Build history of the part. All positions in model axes, mm. A direction names the side the tool comes from. Coordinates: 2 decimals unless noted, no trailing zeros. Order: outer loops, then holes, each group sorted by start corner. A loop starts at its lowest first (then second) coordinate and runs counter-clockwise, first axis right, second up. Notation, with made-up numbers: (-26, 45.5) - (-1, 45.5) arc R32 cw to (-1, 80.5) - close; hole circle Ø11 at (45, 39.25). An arc over 180 degrees is marked (long way). One line per item, written item: value.
from build123d import *
from build123d.topology import SkipClean

# Parameters (mm, degrees)
SKETCH1_R               = 5.5
BOSS_EXTRUDE1_DEPTH     = 17
SKETCH2_R               = 10
BOSS_EXTRUDE2_DEPTH     = 5
BOSS_EXTRUDE3_DEPTH     = 3
BOSS_EXTRUDE4_START     = -6.6383
BOSS_EXTRUDE4_DEPTH     = 6.6383
CIRPATTERN1_COUNT       = 4
SKETCH10_R              = 13.301263659
CUT_EXTRUDE3_DEPTH      = 4
CUT_EXTRUDE3_DEPTH_BACK = 23
FILLET1_R               = 2
CUT_EXTRUDE4_DEPTH      = 6
SKETCH12_R              = 5
CUT_EXTRUDE5_DEPTH      = 3


with BuildPart() as part:
    # Sketch1 → Boss-Extrude1 (new body)
    with BuildSketch(Plane(origin=(0, 0, 0), x_dir=(1, 0, 0), z_dir=(0, 1, 0))):
        with Locations(Location((0, 0, 0), (0, 0, 270))):  # turned: the seam where the file's is
            Circle(SKETCH1_R)
    extrude(amount=BOSS_EXTRUDE1_DEPTH)

    # Sketch2 → Boss-Extrude2 (add)
    with BuildSketch(Plane(origin=(0, 17, 0), x_dir=(1, 0, 0), z_dir=(0, 1, 0))):
        with Locations(Location((0, 0, 0), (0, 0, 270))):  # turned: the seam where the file's is
            Circle(SKETCH2_R)
    extrude(amount=BOSS_EXTRUDE2_DEPTH)

    # Sketch4 → Boss-Extrude3 (add)
    with BuildSketch(Plane(origin=(0, 22, 0), x_dir=(1, 0, 0), z_dir=(0, 1, 0))):
        with BuildLine():
            Line((1, 10), (-1, 10))
            Line((-1, 10), (-1, 4.898979486))
            ThreePointArc((-1, 4.898979486), (-3.535533906, 3.535533906), (-4.898979486, 1))
            Line((-4.898979486, 1), (-10, 1))
            Line((-10, 1), (-10, -1))
            Line((-10, -1), (-4.898979486, -1))
            ThreePointArc((-4.898979486, -1), (-3.535533906, -3.535533906), (-1, -4.898979486))
            Line((-1, -4.898979486), (-1, -10))
            Line((-1, -10), (1, -10))
            Line((1, -10), (1, -4.898979486))
            ThreePointArc((1, -4.898979486), (3.535533906, -3.535533906), (4.898979486, -1))
            Line((4.898979486, -1), (10, -1))
            Line((10, -1), (10, 1))
            Line((10, 1), (4.898979486, 1))
            ThreePointArc((4.898979486, 1), (3.535533906, 3.535533906), (1, 4.898979486))
            Line((1, 4.898979486), (1, 10))
        make_face()
    extrude(amount=BOSS_EXTRUDE3_DEPTH)

    # Sketch9 → Boss-Extrude4 (add)
    with BuildSketch(Plane(origin=(0, 0, -10), x_dir=(-1, 0, 0), z_dir=(0, 0, -1)).offset(BOSS_EXTRUDE4_START)):
        Polygon((-1, 25), (-3.701212133, 22), (-1, 22), align=None)
    boss_extrude4 = extrude(amount=BOSS_EXTRUDE4_DEPTH)

    # CirPattern1: Boss-Extrude4 ×4 about axis
    cirpattern1_axis = Axis((0, 0, 0), (0, 1, 0))
    for i in range(1, CIRPATTERN1_COUNT):
        add(boss_extrude4.rotate(cirpattern1_axis, i * 360 / CIRPATTERN1_COUNT))

    # Sketch10 → Cut-Extrude3 (cut, two sides)
    with BuildSketch(Plane(origin=(0, 22, 0), x_dir=(1, 0, 0), z_dir=(0, 1, 0))) as cut_extrude3_sk:
        Circle(SKETCH10_R)
        with BuildLine():
            ThreePointArc((9.949874371, 1), (9.987460731, 0.500627751), (10, 0))
            ThreePointArc((10, 0), (-8.276838809, -5.611946127), (3.701212133, 9.2898347))
            ThreePointArc((3.701212133, 9.2898347), (7.985510661, 6.019270677), (9.949874371, 1))
        make_face(mode=Mode.SUBTRACT)
    extrude(amount=CUT_EXTRUDE3_DEPTH, mode=Mode.SUBTRACT)
    extrude(cut_extrude3_sk.sketch, amount=-CUT_EXTRUDE3_DEPTH_BACK, mode=Mode.SUBTRACT)

    # Fillet1
    fillet1_edges = [part.edges().sort_by_distance(p)[0] for p in [
        (0, 17, -5.5),
    ]]
    fillet(fillet1_edges, radius=FILLET1_R)

    # Sketch11 → Cut-Extrude4 (cut)
    with SkipClean():  # keep this step's faces unmerged: merging them makes the solid invalid here
        with BuildSketch(Plane.XZ):
            with BuildLine():
                Line((1.650181126, -2.0735), (1.650181126, 2.0735))
                ThreePointArc((1.650181126, 2.0735), (0, 2.65), (-1.650181126, 2.0735))
                Line((-1.650181126, 2.0735), (-1.650181126, -2.0735))
                ThreePointArc((-1.650181126, -2.0735), (0, -2.65), (1.650181126, -2.0735))
            make_face()
        extrude(amount=-CUT_EXTRUDE4_DEPTH, mode=Mode.SUBTRACT)

    # Sketch12 → Cut-Extrude5 (cut)
    with SkipClean():  # keep this step's faces unmerged: merging them makes the solid invalid here
        with BuildSketch(Plane(origin=(0, 25, 0), x_dir=(1, 0, 0), z_dir=(0, 1, 0))):
            Circle(SKETCH12_R)
        extrude(amount=-CUT_EXTRUDE5_DEPTH, mode=Mode.SUBTRACT)


solid = part.part
1. Flat gauge pins, fed straight in: P1, Ø1.5, axis at x = 7.5, y = 24, coming from the -Z side; P2, Ø3.5, axis at y = 3.5, z = -0.5, coming from the +X side; P3, Ø4.5, axis at y = 3.5, z = -0.5, coming from the -X side. Where does each tip first touch, or does it go through?
Values found:
P1: stops at z = -1
P2: stops at x = 5.5
P3: stops at x = -5.5
2. Two-plate mould, pull along X, no slides. Class faces 4 (the face through (-0.02, 2.96, -2.65)), 5 (the face through (-2.33, 23.52, 7.34)), 6 (the face through (7.34, 23.52, 2.33)): pulls with the +X half, pulls with the -X half, needs draft (parallel to the pull), parting line crosses it, or undercut.
Values found:
face 4: undercut
face 5: pulls with the -X half
face 6: needs draft
3. Band-saw the part on C-C, the plane y = 11. Give the cut face in (x, z).
Values found:
outline: circle Ø11 at (0, 0)
4. 3-axis set-ups, long thin cutter, end or side, ignore diameter. For faces 1 (the face through (1, 23, 7)), 2 (the face through (-1, 23, -7)), 3 (the face through (-1.65, 3, 0)): which of +Z, -Z, +X, -X, +Y, -Y reach the whole face in a straight line?
Values found:
face 1: +Z, +X, +Y
face 2: -Z, -X, +Y
face 3: -Y
5. Band-saw the part on B-B, the plane x = 0. Give the cut face in (y, z), and give its area (3 significant figures).
Values found:
outline: (0, -5.5) - (15, -5.5) arc R2 cw to (17, -7.5) - (17, -10) - (25, -10) - (25, -5) - (22, -5) - (22, 5) - (25, 5) - (25, 10) - (17, 10) - (17, 7.5) arc R2 cw to (15, 5.5) - (0, 5.5) - (0, 2.65) - (6, 2.65) - (6, -2.65) - (0, -2.65) - close
area: 287 mm2
6. Band-saw the part on D-D, the plane x = -8.5. Give the cut face in (y, z).
Values found:
outline: (17, -5.27) - (22, -5.27) - (22, -3.7) - (25, -1) - (25, 1) - (22, 1) - (22, 5.27) - (17, 5.27) - close
7. Probe line 1 along Y through (x, z) = (1, -3.5); line 2 along X through (y, z) = (5.5, -0.75); line 3 along Y through (x, z) = (-7.25, -0.5). List the from-to ranges inside material, lowest first.
Values found:
line 1: y = 0 to 22
line 2: x = -5.45 to -1.65, 1.65 to 5.45
line 3: y = 16.99 to 25
8. Band-saw the part on A-A, the plane y = 23. Give the cut face in (x, z).
Values found:
outline: (-9.95, 1) arc R10 ccw to (-9.6, -2.8) - (-4.14, -2.8) arc R5 cw to (-4.9, 1) - close; (-2.8, 4.14) arc R5 cw to (1, 4.9) - (1, 9.95) arc R10 ccw to (-2.8, 9.6) - close; (-1, -9.95) arc R10 ccw to (2.8, -9.6) - (2.8, -4.14) arc R5 cw to (-1, -4.9) - close; (4.14, 2.8) arc R5 cw to (4.9, -1) - (9.95, -1) arc R10 ccw to (9.6, 2.8) - close
